from build123d import *

# Parameters (mm, degrees)
F0_W      = 37.4
F0_H      = 31.4
F0_W_2    = 15.7
F0_H_2    = 2.9
F1_DEPTH  = 147
F2_W      = 37.4
F2_H      = 31.4
F3_DEPTH  = 3
F4_R      = 2
F5_R      = 0.99999
F7_R      = 1.75
F8_DEPTH  = 1
F9_R      = 0.99999
F11_R     = 1.75
F12_DEPTH = 1
F13_R     = 0.99999


# Not quite as in the source:
# - a fillet or chamfer is up to 0.001 mm smaller than in the source, because OpenCascade refuses the exact size


with BuildPart() as f1:
    # F0 (on Front) → F1 (new body)
    with BuildSketch(Plane.XZ):
        with Locations((1, -17.2441455504)):
            Rectangle(F0_W, F0_H)
        with Locations((-7.85, -29.4941455504)):
            Rectangle(F0_W_2, F0_H_2, mode=Mode.SUBTRACT)
        with Locations((-7.85, -24.5941455504)):
            Rectangle(F0_W_2, F0_H_2, mode=Mode.SUBTRACT)
        with Locations((-7.85, -19.6941455504)):
            Rectangle(F0_W_2, F0_H_2, mode=Mode.SUBTRACT)
        with Locations((9.85, -29.4941455504)):
            Rectangle(F0_W_2, F0_H_2, mode=Mode.SUBTRACT)
        with Locations((9.85, -24.5941455504)):
            Rectangle(F0_W_2, F0_H_2, mode=Mode.SUBTRACT)
        with Locations((9.85, -19.6941455504)):
            Rectangle(F0_W_2, F0_H_2, mode=Mode.SUBTRACT)
        with Locations((-7.85, -14.7941455504)):
            Rectangle(F0_W_2, F0_H_2, mode=Mode.SUBTRACT)
        with Locations((-7.85, -9.8941455504)):
            Rectangle(F0_W_2, F0_H_2, mode=Mode.SUBTRACT)
        with Locations((-7.85, -4.9941455504)):
            Rectangle(F0_W_2, F0_H_2, mode=Mode.SUBTRACT)
        with Locations((9.85, -14.7941455504)):
            Rectangle(F0_W_2, F0_H_2, mode=Mode.SUBTRACT)
        with Locations((9.85, -9.8941455504)):
            Rectangle(F0_W_2, F0_H_2, mode=Mode.SUBTRACT)
        with Locations((9.85, -4.9941455504)):
            Rectangle(F0_W_2, F0_H_2, mode=Mode.SUBTRACT)
    extrude(amount=F1_DEPTH)

    # F2 (on face) → F3 (join)
    with BuildSketch(Plane.XZ.offset(147)):
        with Locations((1, -17.2441455504)):
            Rectangle(F2_W, F2_H)
    extrude(amount=F3_DEPTH)

    # F4
    f4_edges = [f1.edges().sort_by_distance(p)[0] for p in [
        (1, -150, -1.544146),
        (-17.7, -150, -17.244146),
        (1, -150, -32.944146),
        (19.7, -150, -17.244146),
    ]]
    fillet(f4_edges, radius=F4_R)

    # F5 (radius 1 in the source; OpenCascade refuses exactly that, so slightly less here)
    f5_edges = [f1.edges().sort_by_distance(p)[0] for p in [
        (1, 0, -1.544146),
        (-17.7, 0, -17.244146),
        (1, 0, -32.944146),
        (19.7, 0, -17.244146),
        (-15.7, 0, -29.494146),
        (-7.85, 0, -28.044146),
        (0, 0, -29.494146),
        (-7.85, 0, -30.944146),
        (-15.7, 0, -24.594146),
        (-7.85, 0, -23.144146),
        (0, 0, -24.594146),
        (-7.85, 0, -26.044146),
        (-15.7, 0, -19.694146),
        (-7.85, 0, -18.244146),
        (0, 0, -19.694146),
        (-7.85, 0, -21.144146),
        (2, 0, -29.494146),
        (9.85, 0, -28.044146),
        (17.7, 0, -29.494146),
        (9.85, 0, -30.944146),
        (2, 0, -24.594146),
        (9.85, 0, -23.144146),
        (17.7, 0, -24.594146),
        (9.85, 0, -26.044146),
        (2, 0, -19.694146),
        (9.85, 0, -18.244146),
        (17.7, 0, -19.694146),
        (9.85, 0, -21.144146),
        (-15.7, 0, -14.794146),
        (-7.85, 0, -13.344146),
        (0, 0, -14.794146),
        (-7.85, 0, -16.244146),
        (-15.7, 0, -9.894146),
        (-7.85, 0, -8.444146),
        (0, 0, -9.894146),
        (-7.85, 0, -11.344146),
        (-15.7, 0, -4.994146),
        (-7.85, 0, -3.544146),
        (0, 0, -4.994146),
        (-7.85, 0, -6.444146),
        (2, 0, -14.794146),
        (9.85, 0, -13.344146),
        (17.7, 0, -14.794146),
        (9.85, 0, -16.244146),
        (2, 0, -9.894146),
        (9.85, 0, -8.444146),
        (17.7, 0, -9.894146),
        (9.85, 0, -11.344146),
        (2, 0, -4.994146),
        (9.85, 0, -3.544146),
        (17.7, 0, -4.994146),
        (9.85, 0, -6.444146),
    ]]
    fillet(f5_edges, radius=F5_R)

    # F7 (on face) → F8 (join)
    with BuildSketch(Plane.XY.offset(-1.5441455504)):
        with Locations((1, -18)):
            Circle(F7_R)
    extrude(amount=F8_DEPTH)

    # F9 (radius 1 in the source; OpenCascade refuses exactly that, so slightly less here)
    f9_edges = [f1.edges().sort_by_distance(p)[0] for p in [
        (-0.75, -18, -0.544146),
    ]]
    fillet(f9_edges, radius=F9_R)

    # F11 (on face) → F12 (join)
    with BuildSketch(Plane(origin=(0, 0, -32.9441455504), x_dir=(1, 0, 0), z_dir=(0, 0, -1))):
        with Locations((1, 18)):
            Circle(F11_R)
    extrude(amount=F12_DEPTH)

    # F13 (radius 1 in the source; OpenCascade refuses exactly that, so slightly less here)
    f13_edges = [f1.edges().sort_by_distance(p)[0] for p in [
        (-0.75, -18, -33.944146),
    ]]
    fillet(f13_edges, radius=F13_R)


solid = f1.part
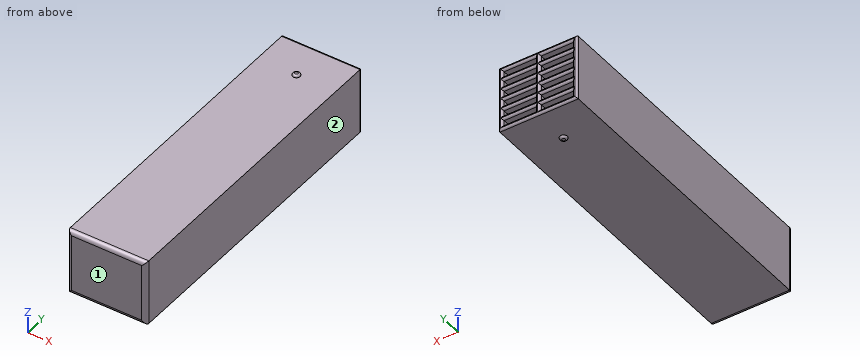
Check sheet for the modelled part. Datum: model origin and axes. Units: mm. Face numbers are marked on the shaded views. Round coordinates to 2 decimals unless told otherwise and drop trailing zeros. One line per item, written item: value. Start each with the question number.
1. Scan lines: line 1 along X through (y, z) = (-21.5, -9.5); line 2 along Y through (x, z) = (-5.5, -16); line 3 along Y through (x, z) = (3, -22.5). Record each from-to range of solid material in increasing order.
2. Section check B-B on y = -41. Give the number of separate pieces and of enclosed holes in the cut face, and give its area (3 significant figures).
3. Release check for a two-part mould opening along Y. For the marked faces 1 and 2 record: released by +Y, released by -Y, zero draft, split by the parting line, or undercut.
4. Gauge pin test, flat ends, axial feed: P1, Ø12.5, axis at x = -11, y = -81, coming from the +Z side; P2, Ø4.5, axis at x = 13.5, y = -54, coming from the -Z side; P3, Ø3, axis at x = -7.5, z = -10, coming from the +Y side; P4, Ø12, axis at x = -6, z = -25, coming from the +Y side. Record the tip position at first contact, or that the pin passes through.
Results found:
1. line 1: -17.7 to -15.7, 0 to 2, 17.7 to 19.7
1. line 2: -150 to -147
1. line 3: -150 to -0.07
2. separate pieces: 1
2. enclosed holes: 12
2. area: 628 mm^2
3. face 1: released by -Y
3. face 2: zero draft
4. P1: z = -1.54
4. P2: z = -32.94
4. P3: y = -0.46
4. P4: y = 0
